The listing builds one solid part. Answer for the finished solid, in the listing's coordinates (mm). A direction names the side the tool comes from. Give positions to 0.01 mm unless a question says otherwise; leave off trailing zeros. Loops run counter-clockwise (first coordinate to the right, second up) from the corner with the lowest first, then second, coordinate; pieces in that order, holes last. Notation, with made-up numbers: (62, -18) - (105, -18) arc R24 cw to (105, 20) - close; hole circle Ø3 at (-27.5, 22). An arc over 180 degrees is marked (long way). Write item = value, one per line. Start each with the question number.
1) Consider probe 1 along X at (y, z) = (0, 1.85); probe 2 along X at (y, z) = (-9, 3.25); probe 3 along X at (y, z) = (-5, -0.4). Determine where each line is inside the solid, lowest interval first.
2) Which of the six approach directions +Z, -Z, +X, -X, +Y, -Y give full straight-line access (tool end or side, diameter ignored) to faces 1 (the cylindrical face through (18.513, 0.195, 1.219)), 2 (the flat face through (-18, -16.2, 0)), 3 (the flat face through (2, -20, 1))?
3) The part is cut by section B-B on y = -21. Write down the section's boundary in (x, z).
4) The part is cut by section C-C on z = 1.6. Write down the section's boundary in (x, y).
5) The part is cut by section D-D on y = 18. Write down the section's boundary in (x, z), plus the area to 3 significant figures.
6) The mould has two halves that part along Z. Classify faces 4 (the cylindrical face through (1.049, 24.478, -0.493)), 5 (the conical face through (-0.643, 15.229, -0.642)), 6 (the flat face through (18, -16.2, 2.5)), 7 (the conical face through (0.643, 15.229, 3.142)): +Z half, -Z half, draft (parallel to the pull), parting line (faces both ways), or undercut.
7) The part is cut by section A-A on y = 0. Write down the section's boundary in (x, z).
8) A flat-ended cylindrical pin translates along its axis: P1, Ø1.4, axis at y = -17.5, z = 1.5, coming from the -X side. Find the tip coordinate at first contact, or state that the pin passes through.
Autodesk Inventor part; units mm, degrees
ref_plane "YZ Plane" through (0, 0, 0) normal (1, 0, 0) x (0, 1, 0)
ref_plane "XZ Plane" through (0, 0, 0) normal (0, 1, 0) x (-1, 0, 0)
ref_plane "XY Plane" through (0, 0, 0) normal (0, 0, 1) x (1, 0, 0)
sketch "Sketch1" plane through (0, 0, 0) normal (0, 0, 1) x (1, 0, 0)
  circle A0 centre (0, 0) radius 15.1
  circle A1 centre (0, 0) radius 24.05
  point P0 (0, 18)
  point P1 (-15.5885, -9)
  point P2 (15.5885, -9)
  dimension "D1" = 30.2
  dimension "d1" = 48.1
  dimension "d2" = 18
  dimension "d5" = 360
extrude "Extrusion1" add sketch "Sketch1" along normal blind 2.5
hole "Hole1" at (0, 18, 0) at (-15.5885, -9, 0) at (15.5885, -9, 0) direction (0, 0, 1) diameter 2 end through all
sketch "Sketch2" plane through (0, 0, 2.5) normal (0, 0, 1) x (1, 0, 0)
  circle A0 centre (0, 0) radius 24.5
  circle A1 centre (0, 18) radius 1
  circle A2 centre (0, 0) radius 15.1
  circle A3 centre (-15.5885, -9) radius 1
  circle A4 centre (15.5885, -9) radius 1
  dimension "d16" = 49
extrude "Extrusion2" add sketch "Sketch2" along normal blind 1
sketch "Sketch3" plane through (0, 0, 0) normal (0, 0, -1) x (-1, 0, 0)
  circle A0 centre (0, 0) radius 24.5
  circle A1 centre (0, 18) radius 1
  circle A2 centre (0, 0) radius 15.1
  circle A3 centre (-15.5885, -9) radius 1
  circle A4 centre (15.5885, -9) radius 1
  dimension "d21" = 49
extrude "Extrusion3" add sketch "Sketch3" along normal blind 1
sketch "Sketch4" plane through (0, 0, 3.5) normal (0, 0, 1) x (1, 0, 0)
  line L0 (2, -30.8109) -> (-2, -30.8109)
  line L1 (-2, -30.8109) -> (-2, -10.8109)
  line L2 (-2, -10.8109) -> (2, -10.8109)
  line L3 (2, -10.8109) -> (2, -30.8109)
  line L4 (2, -30.8109) -> (-2, -10.8109) construction
  line L5 (-2, -30.8109) -> (2, -10.8109) construction
  line L6 (0, -41.8731) -> (0, 35.5622)
  point P0 (0, 0)
  point P1 (0, -20.8109)
  dimension "d22" = 4
  dimension "d23" = 20
  dimension "d33" = 0
extrude "Extrusion4" cut sketch "Sketch4" against normal through all
sketch "Sketch5" plane through (0, 0, 3.5) normal (0, 0, 1) x (1, 0, 0)
  point P0 (0, 0)
  point P1 (-20, 0)
  point P2 (20, 0)
hole "Hole2" at (-20, 0, 3.5) at (20, 0, 3.5) direction (0, 0, -1) diameter 3 end through all
chamfer "Chamfer1" distance 0.5 angle 45 2 edges at (0, 15.1, 3.5) (0, 15.1, -1)
properties part number "Adapter-MitutoyoMT1-SM2-v4(flex)-forDLP"
Answer below:
q1.probe_1 = -24.05 to -21.5, -18.5 to -15.1, 15.1 to 18.5, 21.5 to 24.05
q1.probe_2 = -22.79 to -16.59, -14.59 to -12.43, 12.43 to 14.59, 16.59 to 22.79
q1.probe_3 = -23.98 to -14.25, 14.25 to 23.98
q2.face_1 = +Z, -Z
q2.face_2 = none
q2.face_3 = +Z, -Z, -Y
q3.outline = (-12.62, -1) - (-2, -1) - (-2, 3.5) - (-12.62, 3.5) - (-12.62, 2.5) - (-11.72, 2.5) - (-11.72, 0) - (-12.62, 0) - close; (2, -1) - (12.62, -1) - (12.62, 0) - (11.72, 0) - (11.72, 2.5) - (12.62, 2.5) - (12.62, 3.5) - (2, 3.5) - close
q4.outline = (-2, -23.97) - (-2, -14.97) arc R15.1 cw (long way) to (2, -14.97) - (2, -23.97) arc R24.05 ccw (long way) to start; hole circle Ø3 at (-20, 0); hole circle Ø2 at (-15.59, -9); hole circle Ø2 at (0, 18); hole circle Ø2 at (15.59, -9); hole circle Ø3 at (20, 0)
q5.outline = (-16.62, -1) - (-1, -1) - (-1, 3.5) - (-16.62, 3.5) - (-16.62, 2.5) - (-15.95, 2.5) - (-15.95, 0) - (-16.62, 0) - close; (1, -1) - (16.62, -1) - (16.62, 0) - (15.95, 0) - (15.95, 2.5) - (16.62, 2.5) - (16.62, 3.5) - (1, 3.5) - close
q5.area = 137 mm2
q6.face_4 = draft
q6.face_5 = -Z half
q6.face_6 = undercut
q6.face_7 = +Z half
q7.outline = (-24.5, -1) - (-21.5, -1) - (-21.5, 3.5) - (-24.5, 3.5) - (-24.5, 2.5) - (-24.05, 2.5) - (-24.05, 0) - (-24.5, 0) - close; (-18.5, -1) - (-15.6, -1) - (-15.1, -0.5) - (-15.1, 3) - (-15.6, 3.5) - (-18.5, 3.5) - close; (15.1, -0.5) - (15.6, -1) - (18.5, -1) - (18.5, 3.5) - (15.6, 3.5) - (15.1, 3) - close; (21.5, -1) - (24.5, -1) - (24.5, 0) - (24.05, 0) - (24.05, 2.5) - (24.5, 2.5) - (24.5, 3.5) - (21.5, 3.5) - close
q8.P1 = -17.21
